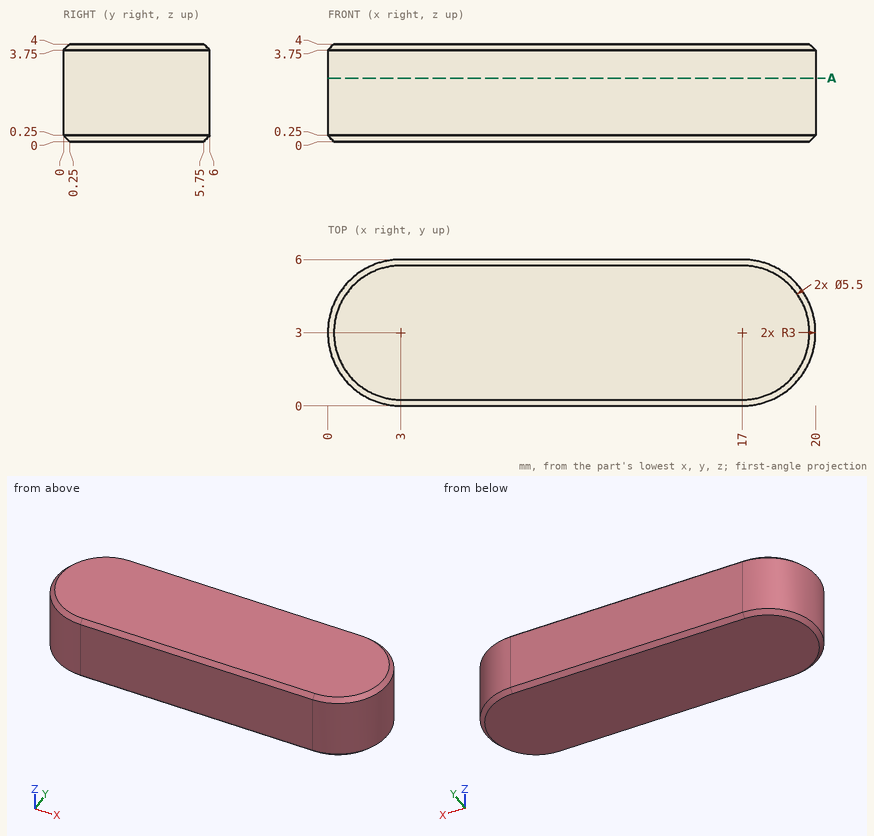
Geometry check sheet. Reference: drawing and pictorial views, mm from the part's lowest x, y, z. Give positions to 0.01 mm unless a question says otherwise; leave off trailing zeros. Loops run counter-clockwise (first coordinate to the right, second up) from the corner with the lowest first, then second, coordinate; pieces in that order, holes last.
1. Section check A-A, the plane z = 2.6. Enter the section's corners in (x, y), then the cut area to 3 significant figures.
2. Go/stop test with a flat-tipped pin: pin 1 Ø1 at (y, z) = (4, 3) entering from +X. Record where the tip stops, or that it passes through.
3. Thickness scan on line 1 (Y direction, x = 19, z = 2.4); line 2 (Y direction, x = 1.75, z = 1.45); line 3 (X direction, y = 0.9, z = 1.3). Record the ranges inside material, lowest first.
Geometry says:
1. outline: (3, 0) - (17, 0) arc R3 ccw to (17, 6) - (3, 6) arc R3 ccw to start
1. area: 112 mm2
2. pin 1: stops at x = 19.96
3. line 1: y = 0.76 to 5.24
3. line 2: y = 0.27 to 5.73
3. line 3: x = 0.86 to 19.14
